from build123d import *

# Parameters (mm, degrees)
IZIM1_W                            = 40
IZIM1_H                            = 30
Y_KSEKLIK_EKSTR_ZYON1_DEPTH        = 15
KES_EKSTR_ZYON1_DEPTH              = 30
M4_TAPA_I_IN_Z_VANA_MATKAB_1_D     = 3.3
M4_TAPA_I_IN_Z_VANA_MATKAB_1_DEPTH = 15
M4_TAPA_I_IN_Z_VANA_MATKAB_1_TIP   = 0.991420021
M4_TAPA_I_IN_Z_VANA_MATKAB_3_D     = 3.3
M4_TAPA_I_IN_Z_VANA_MATKAB_3_DEPTH = 13
M4_TAPA_I_IN_Z_VANA_MATKAB_3_TIP   = 0.991420021


with BuildPart() as part:
    # Çizim1 → Yükseklik-Ekstrüzyon1 (new body, symmetric)
    with BuildSketch(Plane.XY):
        Rectangle(IZIM1_W, IZIM1_H)
    extrude(amount=Y_KSEKLIK_EKSTR_ZYON1_DEPTH, both=True)

    # Çizim2 → Kes-Ekstrüzyon1 (cut)
    with BuildSketch(Plane.XY.offset(15)):
        with BuildLine():
            Line((-6.25, -15), (-6.25, -9.354143467))
            ThreePointArc((-6.25, -9.354143467), (0, 11.25), (6.25, -9.354143467))
            Line((6.25, -9.354143467), (6.25, -15))
            Line((6.25, -15), (-6.25, -15))
        make_face()
    extrude(amount=-KES_EKSTR_ZYON1_DEPTH, mode=Mode.SUBTRACT)

    # M4 Tapa için Zıvana matkabı1
    with Locations(Plane(origin=(-11.313708499, 11.313708499, 15), x_dir=(1, 0, 0), z_dir=(0, 0, 1))):
        with Locations((0, 0), (-4.686291501, -11.313708499), (0, -22.627416998), (22.627416998, -22.627416998), (27.313708499, -11.313708499), (22.627416998, 0)):
            Hole(M4_TAPA_I_IN_Z_VANA_MATKAB_1_D / 2, depth=M4_TAPA_I_IN_Z_VANA_MATKAB_1_DEPTH)
            with Locations((0, 0, -(M4_TAPA_I_IN_Z_VANA_MATKAB_1_DEPTH + M4_TAPA_I_IN_Z_VANA_MATKAB_1_TIP / 2))):  # 118° drill point
                Cone(0, M4_TAPA_I_IN_Z_VANA_MATKAB_1_D / 2, M4_TAPA_I_IN_Z_VANA_MATKAB_1_TIP, mode=Mode.SUBTRACT)

    # M4 Tapa için Zıvana matkabı3
    with Locations(Plane(origin=(-16, 15, -9.5), x_dir=(1, 0, 0), z_dir=(0, 1, 0))):
        with Locations((0, 0), (0, -19), (32, 0), (32, -19)):
            Hole(M4_TAPA_I_IN_Z_VANA_MATKAB_3_D / 2, depth=M4_TAPA_I_IN_Z_VANA_MATKAB_3_DEPTH)
            with Locations((0, 0, -(M4_TAPA_I_IN_Z_VANA_MATKAB_3_DEPTH + M4_TAPA_I_IN_Z_VANA_MATKAB_3_TIP / 2))):  # 118° drill point
                Cone(0, M4_TAPA_I_IN_Z_VANA_MATKAB_3_D / 2, M4_TAPA_I_IN_Z_VANA_MATKAB_3_TIP, mode=Mode.SUBTRACT)


solid = part.part
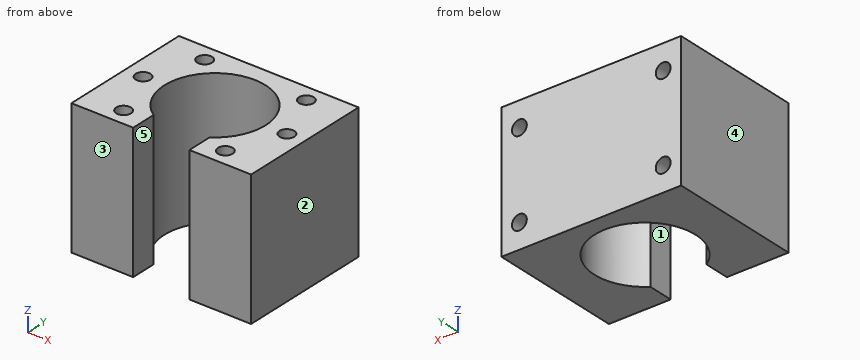
Design review of the part built by this model. Coordinates are the model's own, in mm. Face numbers are marked on the shaded views. A direction names the side the tool comes from. Round coordinates to 2 decimals unless told otherwise and drop trailing zeros. Write each loop counter-clockwise with the first axis right and the second up, starting at its lowest first coordinate (ties: lowest second). Pieces come first, ordered by that corner, then holes.
Item 1: Draft analysis for pull direction X (two halves, no side actions). For the marked faces 1, 2 and 3, state which applies: released by +X, released by -X, zero draft, split by the parting line, or undercut.
Item 2: Consider section D-D on z = 9.5. Give the boundary of the cut face in (x, y), and give its area (3 significant figures).
Item 3: For pin 1 Ø4 at (x, y) = (11.31, 11.31) entering from +Z; pin 2 Ø3 at (x, y) = (16, 0) entering from +Z; pin 3 Ø2 at (x, z) = (0, -9.5) entering from -Y; pin 4 Ø2 at (x, z) = (16, -9.5) entering from +Y, all flat-tipped, find the tip position at first contact; note any pin that passes through.
Item 4: Consider section B-B on y = 4.25. Give the boundary of the cut face in (x, z), and give its area (3 significant figures).
Item 5: Consider section C-C on y = -7. Give the boundary of the cut face in (x, z), and give its area (3 significant figures).
Item 6: Wall thickness on L1, parallel to Y at x = 11.5, z = 2; L2, parallel to X at y = 0, z = 4.75; L3, parallel to Y at x = -16, z = 4.75: over which ranges is each line inside the solid? List them lowest first.
Item 7: For the marked faces 4 and 5, list the 3-axis set-ups (+Z, -Z, +X, -X, +Y, -Y) from which the entire face can be reached by the end or side of a thin tool; tool diameter is ignored.
Item 8: Consider section A-A on x = -9. Give the boundary of the cut face in (y, z), and give its area (3 significant figures).
Check values:
1. face 1: undercut
1. face 2: released by +X
1. face 3: zero draft
2. outline: (-20, -15) - (-6.25, -15) - (-6.25, -9.35) arc R11.25 cw (long way) to (6.25, -9.35) - (6.25, -15) - (20, -15) - (20, 15) - (17.65, 15) - (17.65, 2) - (16.76, 1.46) arc R1.65 cw (long way) to (15.24, 1.46) - (14.35, 2) - (14.35, 15) - (-14.35, 15) - (-14.35, 2) - (-15.24, 1.46) arc R1.65 cw (long way) to (-16.76, 1.46) - (-17.65, 2) - (-17.65, 15) - (-20, 15) - close; hole circle Ø3.3 at (-11.31, -11.31); hole circle Ø3.3 at (-11.31, 11.31); hole circle Ø3.3 at (11.31, -11.31); hole circle Ø3.3 at (11.31, 11.31)
2. area: 609 mm2
3. pin 1: stops at z = 15
3. pin 2: stops at z = -0.09
3. pin 3: stops at y = 11.21
3. pin 4: stops at y = 1.61
4. outline: (-20, -15) - (-10.42, -15) - (-10.42, 15) - (-20, 15) - close; (10.42, -15) - (20, -15) - (20, 15) - (10.42, 15) - close; hole circle Ø3.3 at (-16, -9.5); hole circle Ø3.3 at (-16, 9.5); hole circle Ø3.3 at (16, -9.5); hole circle Ø3.3 at (16, 9.5)
4. area: 541 mm2
5. outline: (-20, -15) - (-8.81, -15) - (-8.81, 15) - (-20, 15) - close; (8.81, -15) - (20, -15) - (20, 15) - (8.81, 15) - close
5. area: 672 mm2
6. L1: y = -15 to -12.95, -9.67 to 9.67, 12.95 to 15
6. L2: x = -20 to -17.65, -14.35 to -11.25, 11.25 to 14.35, 17.65 to 20
6. L3: y = -15 to -1.65, 1.65 to 15
7. face 4: +Z, -Z, -X, +Y, -Y
7. face 5: +Z, -Z, -Y
8. outline: (-15, -15) - (-6.75, -15) - (-6.75, 15) - (-15, 15) - close; (6.75, -15) - (15, -15) - (15, 15) - (6.75, 15) - close
8. area: 495 mm2
